Read the model definition and answer for the solid it produces. Units are mm, in the model's axes. A direction names the side the tool comes from. Coordinates: 2 decimals unless noted, no trailing zeros. Loops run counter-clockwise (first coordinate to the right, second up) from the corner with the lowest first, then second, coordinate; pieces in that order, holes last. Notation, with made-up numbers: (58.5, -6) -> (117.5, -6) arc R16 ccw to (117.5, 3) -> close; hole circle Ø3 at (22.25, -0.5). An arc over 180 degrees is marked (long way). Answer in a Markdown table with one row per item.
Autodesk Inventor part; units mm, degrees
ref_plane "YZ Plane" through (0, 0, 0) normal (1, 0, 0) x (0, 1, 0)
ref_plane "XZ Plane" through (0, 0, 0) normal (0, 1, 0) x (-1, 0, 0)
ref_plane "XY Plane" through (0, 0, 0) normal (0, 0, 1) x (1, 0, 0)
sketch "Sketch1" plane through (0, 0, 0) normal (0, 1, 0) x (-1, 0, 0)
  line L0 (60.75, -57.25) -> (-60.75, -57.25)
  line L1 (-60.75, -57.25) -> (-60.75, 57.25)
  line L2 (-60.75, 57.25) -> (60.75, 57.25)
  line L3 (60.75, 57.25) -> (60.75, -57.25)
  line L4 (0, -80.15) -> (0, 80.15)
  line L5 (-85.05, 0) -> (85.05, 0)
  dimension "d0" = 121.5
  dimension "d1" = 114.5
extrude "Extrusion1" add sketch "Sketch1" along normal blind 5
sketch "Sketch3" plane through (0, 5, 0) normal (0, 1, 0) x (1, 0, 0)
  circle A0 centre (-36.75, -34.25) radius 1.5
  line L0 (-60.75, 57.25) -> (-60.75, -57.25)
  circle A1 centre (-12.75, -34.25) radius 1.5
  circle A2 centre (-36.75, -42.25) radius 1.5
  circle A3 centre (-12.75, -42.25) radius 1.5
  line L1 (-60.75, -57.25) -> (60.75, -57.25)
  circle A4 centre (-55.75, -22.25) radius 1.5
  circle A5 centre (-55.75, 17.75) radius 1.5
  circle A6 centre (-25.25, 51.25) radius 1.5
  circle A7 centre (28.75, 51.25) radius 1.5
  circle A8 centre (55.75, 17.75) radius 1.5
  circle A9 centre (55.75, -22.25) radius 1.5
  line L2 (60.75, 57.25) -> (-60.75, 57.25)
  line L3 (60.75, -57.25) -> (60.75, 57.25)
  circle A10 centre (-25.25, -10.75) radius 1.5
  circle A11 centre (28.75, -10.75) radius 1.5
  circle A12 centre (6.75, -29.75) radius 1.5
  circle A13 centre (6.75, -48.75) radius 1.5
  circle A14 centre (35.75, -48.75) radius 1.5
  circle A15 centre (35.75, -29.75) radius 1.5
  point P0 (0, 0)
  dimension "d11" = 3
  dimension "d12" = 24
  dimension "d13" = 3
  dimension "d14" = 3
  dimension "d15" = 3
  dimension "d16" = 24
  dimension "d17" = 24
  dimension "d20" = 23
  dimension "d21" = 23
  dimension "d22" = 8
  dimension "d23" = 8
  dimension "d24" = 15
  dimension "d25" = 3
  dimension "d26" = 3
  dimension "d27" = 5
  dimension "d28" = 5
  dimension "d29" = 35
  dimension "d30" = 40
  dimension "d31" = 3
  dimension "d32" = 3
  dimension "d33" = 3
  dimension "d34" = 3
  dimension "d35" = 6
  dimension "d36" = 6
  dimension "d37" = 5
  dimension "d38" = 5
  dimension "d39" = 35
  dimension "d40" = 40
  dimension "d41" = 32
  dimension "d42" = 54
  dimension "d43" = 3
  dimension "d44" = 3
  dimension "d45" = 62
  dimension "d46" = 62
  dimension "d47" = 54
  dimension "d48" = 32
  dimension "d49" = 3
  dimension "d50" = 3
  dimension "d51" = 3
  dimension "d52" = 3
  dimension "d53" = 8.5
  dimension "d54" = 8.5
  dimension "d55" = 25
  dimension "d56" = 29
  dimension "d57" = 19
  dimension "d58" = 19
  dimension "d59" = 25
  dimension "d60" = 29
extrude "Extrusion2" cut sketch "Sketch3" against normal through all contours A0 | A1 | A2 | A3 | A4 | A5 | A6 | A7 | A8 | A9 | A10 | A11 | A12 | A13 | A14 | A15
sketch "Sketch4" plane through (0, 5, 0) normal (0, 1, 0) x (1, 0, 0)
  line L0 (-44.75, -29.25) -> (-6.75, -29.25)
  line L1 (-6.75, -29.25) -> (-6.75, -46.25)
  line L2 (-6.75, -46.25) -> (-44.75, -46.25)
  line L3 (-44.75, -46.25) -> (-44.75, -29.25)
  line L4 (-50.75, -25.25) -> (-1.75, -25.25)
  line L5 (-1.75, -25.25) -> (-1.75, -53.25)
  line L6 (-1.75, -53.25) -> (-50.75, -53.25)
  line L7 (-50.75, -53.25) -> (-50.75, -25.25)
  line L8 (-60.75, 57.25) -> (-60.75, -57.25)
  line L9 (-60.75, -57.25) -> (60.75, -57.25)
  circle A0 centre (6.75, -29.75) radius 1.5
  circle A1 centre (6.75, -29.75) radius 4
  circle A2 centre (6.75, -29.75) radius 6
  circle A3 centre (6.75, -48.75) radius 1.5
  circle A4 centre (6.75, -48.75) radius 4
  circle A5 centre (6.75, -48.75) radius 6
  circle A6 centre (35.75, -29.75) radius 1.5
  circle A7 centre (35.75, -29.75) radius 4
  circle A8 centre (35.75, -29.75) radius 6
  circle A9 centre (35.75, -48.75) radius 1.5
  circle A10 centre (35.75, -48.75) radius 4
  circle A11 centre (35.75, -48.75) radius 6
  circle A12 centre (28.75, -10.75) radius 1.5
  circle A13 centre (28.75, -10.75) radius 4
  circle A14 centre (28.75, -10.75) radius 6
  circle A15 centre (-25.25, -10.75) radius 1.5
  circle A16 centre (-25.25, -10.75) radius 4
  circle A17 centre (-25.25, -10.75) radius 6
  circle A18 centre (-25.25, 51.25) radius 1.5
  circle A19 centre (-25.25, 51.25) radius 4
  circle A20 centre (-25.25, 51.25) radius 6
  circle A21 centre (28.75, 51.25) radius 1.5
  circle A22 centre (28.75, 51.25) radius 4
  circle A23 centre (28.75, 51.25) radius 6
  point P0 (0, 0)
  dimension "d63" = 49
  dimension "d64" = 28
  dimension "d71" = 5
  dimension "d72" = 4
  dimension "d73" = 6
  dimension "d74" = 7
  dimension "d75" = 59
  dimension "d76" = 32
  dimension "d77" = 8
  dimension "d78" = 12
  dimension "d79" = 8
  dimension "d80" = 12
  dimension "d81" = 8
  dimension "d82" = 12
  dimension "d83" = 8
  dimension "d84" = 12
  dimension "d85" = 8
  dimension "d86" = 12
  dimension "d87" = 8
  dimension "d88" = 12
  dimension "d89" = 8
  dimension "d90" = 12
  dimension "d91" = 8
  dimension "d92" = 12
extrude "Extrusion3" add sketch "Sketch4" along normal blind 4 contours L4 L5 L6 L7 | A2 | A5 | A8 | A11 | A14 | A17 | A20 | A23
properties part number "circuirt_board"
1. A cutting plane is placed at C-C on z = 22.25. Give the vertices of the cut face in (x, y).
A:
| item | result |
|---|---|
| outline | (-60.75, 0) -> (-57.25, 0) -> (-57.25, 5) -> (-60.75, 5) -> close; (-54.25, 0) -> (54.25, 0) -> (54.25, 5) -> (-54.25, 5) -> close; (57.25, 0) -> (60.75, 0) -> (60.75, 5) -> (57.25, 5) -> close |
2. A cutting plane is placed at D-D on x = -36.75. Give the vertices of the cut face in (y, z).
A:
| item | result |
|---|---|
| outline | (0, -57.25) -> (5, -57.25) -> (5, 25.25) -> (9, 25.25) -> (9, 29.25) -> (5, 29.25) -> (5, 32.75) -> (0, 32.75) -> close; (0, 35.75) -> (5, 35.75) -> (5, 40.75) -> (0, 40.75) -> close; (0, 43.75) -> (5, 43.75) -> (5, 46.25) -> (9, 46.25) -> (9, 53.25) -> (5, 53.25) -> (5, 57.25) -> (0, 57.25) -> close |
3. A tool of negligible diameter and unlimited length cuts with its end or side. For faces 4 (the flat face through (7, 5, 28)), 5 (the flat face through (-27, 9, 48)), from which of +Z, -Z, +X, -X, +Y, -Y can it reach the whole face along a straight path? Write none if from no direction.
A:
| item | result |
|---|---|
| face 4 | +Y |
| face 5 | +Z, -Z, +X, -X, +Y |
4. A cutting plane is placed at A-A on y = 7.5. Count the separate pieces of the cut face and the enclosed holes in it, and give its area (3 significant figures).
A:
| item | result |
|---|---|
| separate pieces | 9 |
| enclosed holes | 9 |
| area | 1,230 mm2 |
5. The mould has two halves that part along Z. Classify faces 1 (the flat face through (-26, 7, 53.25)), 2 (the flat face through (-50.75, 7, 39)), 3 (the cylindrical face through (6.229, 6.972, 33.716)): pulls with the +Z half, pulls with the -Z half, needs draft (parallel to the pull), parting line crosses it, or undercut.
A:
| item | result |
|---|---|
| face 1 | pulls with the +Z half |
| face 2 | needs draft |
| face 3 | undercut |
6. A cutting plane is placed at B-B on x = -55.75. Give the vertices of the cut face in (y, z).
A:
| item | result |
|---|---|
| outline | (0, -57.25) -> (5, -57.25) -> (5, -19.25) -> (0, -19.25) -> close; (0, -16.25) -> (5, -16.25) -> (5, 20.75) -> (0, 20.75) -> close; (0, 23.75) -> (5, 23.75) -> (5, 57.25) -> (0, 57.25) -> close |
7. Find the intervals of material crossed by probe 1 along Z at (x, y) = (-25.25, 6.1); probe 2 along Z at (x, y) = (-55.75, 3.6); probe 3 along X at (y, z) = (6.75, -51.25), in increasing order.
A:
| item | result |
|---|---|
| probe 1 | z = -57.25 to -55.25, -47.25 to -45.25, 4.75 to 6.75, 14.75 to 16.75, 25.25 to 29.25, 46.25 to 53.25 |
| probe 2 | z = -57.25 to -19.25, -16.25 to 20.75, 23.75 to 57.25 |
| probe 3 | x = -31.25 to -29.25, -21.25 to -19.25, 22.75 to 24.75, 32.75 to 34.75 |
8. Given pin 1 Ø3 at (y, z) = (7, -1.5) entering from +X; pin 2 Ø7 at (x, z) = (6.75, 48.75) entering from -Y; pin 3 Ø1.2 at (x, y) = (-30.5, 7) entering from -Z; pin 4 Ø6.5 at (x, z) = (35.75, 48.75) entering from +Y, each flat-ended and moving along its own axis, determine where each tip first touches the part or whether it passes through.
A:
| item | result |
|---|---|
| pin 1 | passes through |
| pin 2 | stops at y = 0 |
| pin 3 | stops at z = -55.04 |
| pin 4 | stops at y = 5 |
